Autodesk Inventor part; units mm, degrees
ref_plane "YZ Plane" through (0, 0, 0) normal (1, 0, 0) x (0, 1, 0)
ref_plane "XZ Plane" through (0, 0, 0) normal (0, 1, 0) x (-1, 0, 0)
ref_plane "XY Plane" through (0, 0, 0) normal (0, 0, 1) x (1, 0, 0)
sketch "Sketch1" plane through (0, 0, 0) normal (0, 1, 0) x (-1, 0, 0)
  circle A0 centre (0, 0) radius 1.5
  dimension "d0" = 3
extrude "Extrusion1" add sketch "Sketch1" along normal blind 6
sketch "Sketch2" plane through (0, 6, 0) normal (0, 1, 0) x (1, 0, 0)
  circle A0 centre (0, 0) radius 2.5
  dimension "d3" = 5
extrude "Extrusion2" add sketch "Sketch2" along normal blind 2
fillet "Fillet1" radius 1.7 1 edges at (-2.5, 8, 0)
chamfer "Chamfer1" distance 0.3 angle 45 1 edges at (1.5, 0, 0)
thread "Thread1"
sketch "Sketch3" plane through (0, 8, 0) normal (0, 1, 0) x (1, 0, 0)
  line L0 (0.5, -2.5) -> (0.5, 2.5)
  line L1 (0.5, 2.5) -> (-0.5, 2.5)
  line L2 (-0.5, 2.5) -> (-0.5, -2.5)
  line L3 (-0.5, -2.5) -> (0.5, -2.5)
  line L4 (0.5, -2.5) -> (-0.5, 2.5) construction
  line L5 (0.5, 2.5) -> (-0.5, -2.5) construction
  line L6 (1.5, -0.5) -> (-1.5, -0.5)
  line L7 (-1.5, -0.5) -> (-1.5, 0.5)
  line L8 (-1.5, 0.5) -> (1.5, 0.5)
  line L9 (1.5, 0.5) -> (1.5, -0.5)
  circle A0 centre (0, 0) radius 2.5
  line L10 (1.5, -0.5) -> (-1.5, 0.5) construction
  line L11 (-1.5, -0.5) -> (1.5, 0.5) construction
  dimension "d12" = 1
  dimension "d13" = 3
  dimension "d14" = 1
extrude "Extrusion3" cut sketch "Sketch3" against normal blind 0.7 contours L3 A0 L0 | A0 L2 L6 L0 | L3 L2 A0 | L6 L2 L8 L0 | L0 L8 L9 L6 | L8 L2 A0 L0 | L6 L7 L8 L2 | A0 L1 L0 | L2 L1 A0
properties part number "M3x10 Screw Nylon" material "Steel"
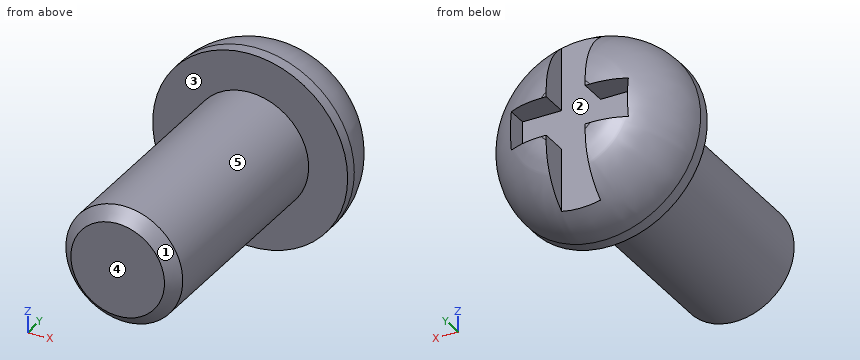
Verification items for the finished model (mm, model axes). Face numbers are marked on the shaded views. A direction names the side the tool comes from. Coordinates: 2 decimals unless noted, no trailing zeros. Write each loop counter-clockwise with the first axis right and the second up, starting at its lowest first coordinate (ties: lowest second). Pieces come first, ordered by that corner, then holes. Notation, with made-up numbers: M 56.25,-28.75 L 97.25,-28.75 A26 cw 97.25,-5.75 Z; hole C -24.75,-26 d3. An arc over 180 degrees is marked long. Answer as a JSON object with one key per item and string values. Group by question number.
(1) Tool access check on the marked faces 4 and 5. Record the directions out of +Z, -Z, +X, -X, +Y, -Y that give a thin tool (end or side, any length) a straight path to the whole face; none if there is none.
(2) Gauge pin test, flat ends, axial feed: pin 1 (0.6 mm diameter, centred on y = 7.5, z = 0, fed in from -X); pin 2 (0.6 mm diameter, centred on x = -1, y = 8, fed in from +Z); pin 3 (0.6 mm diameter, centred on y = 8, z = 1, fed in from -X); pin 4 (0.9 mm diameter, centred on x = 0.5, z = 1, fed in from +Y). Record the tip position at first contact, or that the pin passes through.
(3) Release check for a two-part mould opening along Z. For the marked faces 1, 2 and 3 record: +Z half, -Z half, draft (parallel to the pull), parting line (faces both ways), or undercut.
(4) Cross-section at A-A, the plane y = 1.5. Record the cut outline in (x, z).
(5) Material ranges on line 1 (Y direction, x = 0, z = 0.85); line 2 (X direction, y = 4, z = 0.95); line 3 (Y direction, x = 1.95, z = -0.45), recorded low to high.
Reply:
{
 "1": {"face 4": "+Z, -Z, +X, -X, -Y", "face 5": "-Y"},
 "2": {"pin 1": "x = -2.24", "pin 2": "z = 1.49", "pin 3": "x = -1.49", "pin 4": "y = 8"},
 "3": {"face 1": "parting line", "face 2": "undercut", "face 3": "draft"},
 "4": {"outline": "C 0,0 d3"},
 "5": {"line 1": "0 to 7.3", "line 2": "-1.16 to 1.16", "line 3": "6 to 7.5"}
}
